Read the model definition and answer for the solid it produces. Units are mm, in the model's axes. Face numbers are marked on the shaded views. A direction names the side the tool comes from. Coordinates: 2 decimals unless noted, no trailing zeros. Write each loop counter-clockwise with the first axis right and the second up, starting at its lowest first coordinate (ties: lowest second). Pieces come first, ordered by that corner, then holes. Notation, with made-up numbers: (68, 42.25) - (97, 42.25) arc R28 ccw to (97, 74.25) - close; hole circle Ø11 at (13.5, 42.25). An arc over 180 degrees is marked (long way). Return JSON: item names as keys, results as strings.
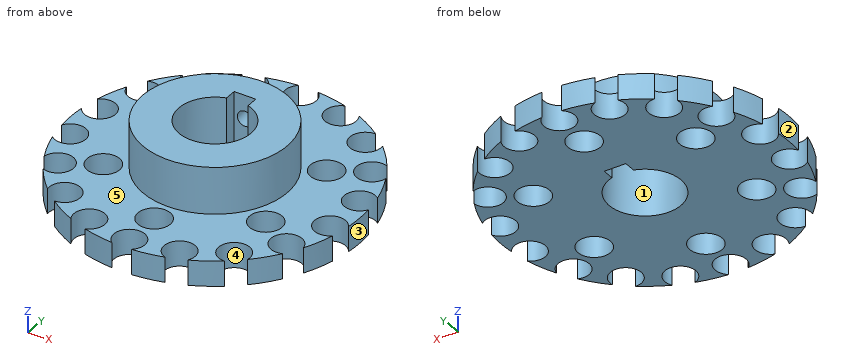
```python
from build123d import *

# Parameters (mm, degrees)
SKETCH_1_R          = 40
EXTRUDE_1_DEPTH     = 7
SKETCH_2_R          = 20
EXTRUDE_2_DEPTH     = 13
SKETCH_3_R          = 4.3
CUT_EXTRUDE_1_DEPTH = 61
SKETCH_4_R          = 4.5
CUT_EXTRUDE_2_DEPTH = 60.938740302
SKETCH_5_R          = 10
CUT_EXTRUDE_3_DEPTH = 60.938740302
SKETCH_6_W          = 6
SKETCH_6_H          = 12.8
CUT_EXTRUDE_4_DEPTH = 60.938740302
SKETCH_8_R          = 2.1
CUT_EXTRUDE_6_DEPTH = 10


with BuildPart() as part:
    # 草图1 → 凸台-拉伸1 (new body)
    with BuildSketch(Plane.XY):
        Circle(SKETCH_1_R)
    extrude(amount=EXTRUDE_1_DEPTH)

    # 草图2 → 凸台-拉伸2 (add)
    with BuildSketch(Plane.XY.offset(7)):
        with Locations(Location((0, 0, 0), (0, 0, 180))):
            Circle(SKETCH_2_R)
    extrude(amount=EXTRUDE_2_DEPTH)

    # 草图3 → 切除-拉伸1 (cut, through all)
    with BuildSketch(Plane.XY):
        with Locations((0, 36.57)):
            Circle(SKETCH_3_R)
        with Locations((-12.507677, 34.364559)):
            Circle(SKETCH_3_R)
        with Locations((-23.506743, 28.014245)):
            Circle(SKETCH_3_R)
        with Locations((-31.670549, 18.285)):
            Circle(SKETCH_3_R)
        with Locations((-36.01442, 6.350314)):
            Circle(SKETCH_3_R)
        with Locations((-36.01442, -6.350314)):
            Circle(SKETCH_3_R)
        with Locations((-31.670549, -18.285)):
            Circle(SKETCH_3_R)
        with Locations((-23.506743, -28.014245)):
            Circle(SKETCH_3_R)
        with Locations((-12.507677, -34.364559)):
            Circle(SKETCH_3_R)
        with Locations((0, -36.57)):
            Circle(SKETCH_3_R)
        with Locations((12.507677, -34.364559)):
            Circle(SKETCH_3_R)
        with Locations((23.506743, -28.014245)):
            Circle(SKETCH_3_R)
        with Locations((31.670549, -18.285)):
            Circle(SKETCH_3_R)
        with Locations((36.01442, -6.350314)):
            Circle(SKETCH_3_R)
        with Locations((36.01442, 6.350314)):
            Circle(SKETCH_3_R)
        with Locations((31.670549, 18.285)):
            Circle(SKETCH_3_R)
        with Locations((23.506743, 28.014245)):
            Circle(SKETCH_3_R)
        with Locations((12.507677, 34.364559)):
            Circle(SKETCH_3_R)
    extrude(amount=CUT_EXTRUDE_1_DEPTH, mode=Mode.SUBTRACT)

    # 草图4 → 切除-拉伸2 (cut, through all)
    with BuildSketch(Plane.XY):
        with Locations((0, 26)):
            Circle(SKETCH_4_R)
        with Locations((-22.51666, 13)):
            Circle(SKETCH_4_R)
        with Locations((-22.51666, -13)):
            Circle(SKETCH_4_R)
        with Locations((0, -26)):
            Circle(SKETCH_4_R)
        with Locations((22.51666, -13)):
            Circle(SKETCH_4_R)
        with Locations((22.51666, 13)):
            Circle(SKETCH_4_R)
    extrude(amount=CUT_EXTRUDE_2_DEPTH, mode=Mode.SUBTRACT)

    # 草图5 → 切除-拉伸3 (cut, through all)
    with BuildSketch(Plane.XY):
        Circle(SKETCH_5_R)
    extrude(amount=CUT_EXTRUDE_3_DEPTH, mode=Mode.SUBTRACT)

    # 草图6 → 切除-拉伸4 (cut, through all)
    with BuildSketch(Plane.XY):
        with Locations((0, 6.4)):
            Rectangle(SKETCH_6_W, SKETCH_6_H)
    extrude(amount=CUT_EXTRUDE_4_DEPTH, mode=Mode.SUBTRACT)

    # 草图8 → 切除-拉伸6 (cut, symmetric)
    with BuildSketch(Plane(origin=(0, 13.5, 0), x_dir=(1, 0, 0), z_dir=(0, 1, 0))):
        with Locations(Location((0, -13.5, 0), (0, 0, 270))):
            Circle(SKETCH_8_R)
    extrude(amount=CUT_EXTRUDE_6_DEPTH, both=True, mode=Mode.SUBTRACT)


solid = part.part
```
(1) A cutting plane is placed at C-C (z = 18.25). Determine the outline of the cut face in (x, y), and give its area (3 significant figures).
Answer:
{"outline": "circle Ø40 at (0, 0); hole (-3, 9.54) arc R10 ccw (long way) to (3, 9.54) - (3, 12.8) - (-3, 12.8) - close", "area": "925 mm²"}
(2) Straight lines are drawn through the part: line 1 (Z direction, x = 0, y = 16.75); line 2 (Y direction, x = -34.5, z = 2); line 3 (Y direction, x = -23, z = 6.25). For each, find the intervals that lie inside material, in ascending order. Write a range as from..to.
Answer:
{"line 1": "0..11.4, 15.6..20", "line 2": "-15.05..-10.37, -2.33..2.33, 10.37..15.05", "line 3": "-32.73..-32.28, -23.74..-17.47, -8.53..8.53, 17.47..23.74, 32.28..32.73"}
(3) A cutting plane is placed at A-A (y = 0). Determine the outline of the cut face in (x, z), and give its area (3 significant figures).
Answer:
{"outline": "(-40, 0) - (-10, 0) - (-10, 20) - (-20, 20) - (-20, 7) - (-40, 7) - close; (10, 0) - (40, 0) - (40, 7) - (20, 7) - (20, 20) - (10, 20) - close", "area": "680 mm²"}
(4) Flat-ended cylindrical pins translate along their axes: P1, Ø8, axis at x = -8.5, z = 6.5, coming from the +Y side; P2, Ø6.5, axis at x = 0, z = 13.5, coming from the +Y side; P3, Ø6, axis at x = -30, y = 2, coming from the +Z side. Find the tip coordinate at first contact, or state that the pin passes through.
Answer:
{"P1": "y = 39.75", "P2": "y = 20", "P3": "z = 7"}
(5) A cutting plane is placed at D-D (y = -13). Determine the outline of the cut face in (x, z), and give its area (3 significant figures).
Answer:
{"outline": "(-37.83, 0) - (-27.02, 0) - (-27.02, 7) - (-37.83, 7) - close; (-18.02, 0) - (18.02, 0) - (18.02, 7) - (15.2, 7) - (15.2, 20) - (-15.2, 20) - (-15.2, 7) - (-18.02, 7) - close; (27.02, 0) - (37.83, 0) - (37.83, 7) - (27.02, 7) - close", "area": "799 mm²"}
(6) Determine the mould class of the marked faces 1, 2 and 3 for opening direction X: +X half, -X half, draft (parallel to the pull), parting line (faces both ways), or undercut.
Answer:
{"face 1": "undercut", "face 2": "-X half", "face 3": "+X half"}
(7) Which of the six approach directions +Z, -Z, +X, -X, +Y, -Y give full straight-line access (tool end or side, diameter ignored) to the marked faces 4 and 5?
Answer:
{"face 4": "+Z, -Z", "face 5": "+Z"}
(8) A cutting plane is placed at B-B (x = 0). Determine the outline of the cut face in (y, z).
Answer:
{"outline": "(-32.27, 0) - (-30.5, 0) - (-30.5, 7) - (-32.27, 7) - close; (-21.5, 0) - (-10, 0) - (-10, 20) - (-20, 20) - (-20, 7) - (-21.5, 7) - close; (12.8, 0) - (21.5, 0) - (21.5, 7) - (20, 7) - (20, 11.4) - (12.8, 11.4) - close; (12.8, 15.6) - (20, 15.6) - (20, 20) - (12.8, 20) - close; (30.5, 0) - (32.27, 0) - (32.27, 7) - (30.5, 7) - close"}
